Source: CAD feature listing. Evaluate the final solid. Frame: model axes, mm. A direction names the side the tool comes from. Coordinates: 2 decimals unless noted, no trailing zeros. Loops run counter-clockwise (first coordinate to the right, second up) from the corner with the lowest first, then second, coordinate; pieces in that order, holes last.
```python
from build123d import *

# Parameters (mm, degrees)
BOSS_EXTRUDE1_DEPTH      = 48
BOSS_EXTRUDE1_DEPTH_BACK = 1
SKETCH1_R                = 28.506
SKETCH1_R_2              = 27.506
CUT_EXTRUDE1_DEPTH       = 48


with BuildPart() as part:
    # Sketch1 → Boss-Extrude1 (new, two sides: drawn at the far end of the back side and taken through both)
    with BuildSketch(Plane(origin=(0, 0, 0), x_dir=(1, 0, 0), z_dir=(0, 1, 0)).offset(-BOSS_EXTRUDE1_DEPTH_BACK)):
        with Locations(Location((0, 0, 0), (0, 0, 270))):
            Circle(SKETCH1_R)
        with Locations(Location((0, 0, 0), (0, 0, 270))):
            Circle(SKETCH1_R_2, mode=Mode.SUBTRACT)
    extrude(amount=BOSS_EXTRUDE1_DEPTH + BOSS_EXTRUDE1_DEPTH_BACK)

    # Sketch2 → Cut-Extrude1 (cut)
    with BuildSketch(Plane(origin=(0, 0, 0), x_dir=(0, 0, -1), z_dir=(1, 0, 0))):
        with BuildLine():
            Line((11.666, 18.5), (11.666, 48))
            Line((11.666, 48), (-11.666, 48))
            Line((-11.666, 48), (-11.666, 18.5))
            ThreePointArc((-11.666, 18.5), (0, 6.834), (11.666, 18.5))
        make_face()
    extrude(amount=-CUT_EXTRUDE1_DEPTH, mode=Mode.SUBTRACT)


solid = part.part
```
Q1. Section query B-B on x = 0. Return the cut outline in (y, z).
Q2. Section query A-A on z = 0. Return the cut outline in (x, y).
Q3. Draft query along X for faces 1 (the flat face through (18, 48, -21)), 2 (the cylindrical face through (27.272, 23.157, -3.581)), 3 (the cylindrical face through (24.04, 23.16, 15.32)). Return one class per face: released by +X, released by -X, zero draft, split by the parting line, or undercut.
Q4. Reachability of faces 4 (the flat face through (23.4, -1, -14.9)), 5 (the cylindrical face through (-27.765, 6.834, 0.086)) from +Z, -Z, +X, -X, +Y, -Y: full face, straight path, thin tool, end or side. Return the list, or none.
Q5. Material intervals for line 1 along Z through (x, y) = (0, 21); line 2 along X through (y, z) = (20.5, 0); line 3 along Z through (x, y) = (9.5, 33), sorted ascending.
Q6. First-contact query: pin 1 Ø10 at (x, y) = (9, 34.5) entering from -Z; pin 2 Ø1 at (y, z) = (24, -13) entering from -X; pin 3 Ø5 at (x, y) = (-17.5, 17) entering from +Z. Flat tips, straight axial feed; report the tip coordinate or a pass-through.
Q7. Section query C-C on y = 4.5. Return the cut outline in (x, z).
Q8. Section query D-D on y = 22.5. Return the cut outline in (x, z).
Resolved:
1. outline: (-1, -28.51) - (48, -28.51) - (48, -27.51) - (-1, -27.51) - close; (-1, 27.51) - (48, 27.51) - (48, 28.51) - (-1, 28.51) - close
2. outline: (-28.51, -1) - (-27.51, -1) - (-27.51, 6.83) - (-28.51, 6.83) - close; (27.51, -1) - (28.51, -1) - (28.51, 48) - (27.51, 48) - close
3. face 1: zero draft
3. face 2: undercut
3. face 3: split by the parting line
4. face 4: +Z, -Z, +X, -X, -Y
4. face 5: -X, +Y
5. line 1: z = -28.51 to -27.51, 27.51 to 28.51
5. line 2: x = 27.51 to 28.51
5. line 3: z = -26.88 to -25.81, 25.81 to 26.88
6. pin 1: stops at z = -28.22
6. pin 2: stops at x = -25.62
6. pin 3: stops at z = 24.24
7. outline: circle Ø57.01 at (0, 0); hole circle Ø55.01 at (0, 0)
8. outline: (-26.01, -11.67) arc R28.51 ccw (long way) to (-26.01, 11.67) - (-24.91, 11.67) arc R27.51 cw (long way) to (-24.91, -11.67) - close
